```python
from build123d import *

# Parameters (mm, degrees)
SKETCH1_R               = 22
SKETCH1_R_2             = 20
BOSS_EXTRUDE1_DEPTH     = 40
CUT_EXTRUDE1_DEPTH      = 23
CUT_EXTRUDE1_DEPTH_BACK = 23
BOSS_EXTRUDE2_DEPTH     = 20
SKETCH4_W               = 28
SKETCH4_H               = 39
CUT_EXTRUDE2_DEPTH      = 32
SKETCH5_R               = 3.5
CUT_EXTRUDE3_DEPTH      = 8.79196205
CUT_EXTRUDE3_DEPTH_BACK = 37.20803795
FILLET1_R               = 8


with BuildPart() as part:
    # Sketch1 → Boss-Extrude1 (new body)
    with BuildSketch(Plane(origin=(0, 0, 0), x_dir=(1, 0, 0), z_dir=(0, 1, 0))):
        Circle(SKETCH1_R)
        Circle(SKETCH1_R_2, mode=Mode.SUBTRACT)
    extrude(amount=BOSS_EXTRUDE1_DEPTH)

    # Sketch2 → Cut-Extrude1 (cut, two sides)
    with BuildSketch(Plane.XY) as cut_extrude1_sk:
        Polygon((22, 33), (-22, 0), (22, 0), align=None)
    extrude(amount=CUT_EXTRUDE1_DEPTH, mode=Mode.SUBTRACT)
    extrude(cut_extrude1_sk.sketch, amount=-CUT_EXTRUDE1_DEPTH_BACK, mode=Mode.SUBTRACT)

    # Sketch3 → Boss-Extrude2 (add)
    with BuildSketch(Plane(origin=(-31, 0, 0), x_dir=(0, 0, -1), z_dir=(1, 0, 0))):
        Polygon((14.20803795, 40), (-17.79196205, 40), (-17.79196205, -1), (-15.79196205, -1), (-15.79196205, 1), (-15.79196205, 38), (12.20803795, 38), (12.20803795, 1), (12.20803795, -1), (14.20803795, -1), align=None)
    extrude(amount=BOSS_EXTRUDE2_DEPTH)

    # Sketch4 → Cut-Extrude2 (cut, through all)
    with BuildSketch(Plane(origin=(0, 0, 0), x_dir=(0, 0, -1), z_dir=(1, 0, 0))):
        with Locations((-1.79196205, 18.5)):
            Rectangle(SKETCH4_W, SKETCH4_H)
    extrude(amount=-CUT_EXTRUDE2_DEPTH, mode=Mode.SUBTRACT)

    # Sketch5 → Cut-Extrude3 (cut, two sides)
    with BuildSketch(Plane(origin=(0, 0, -14.20803795), x_dir=(-1, 0, 0), z_dir=(0, 0, -1))) as cut_extrude3_sk:
        with Locations((24, 6)):
            Circle(SKETCH5_R)
    extrude(amount=CUT_EXTRUDE3_DEPTH, mode=Mode.SUBTRACT)
    extrude(cut_extrude3_sk.sketch, amount=-CUT_EXTRUDE3_DEPTH_BACK, mode=Mode.SUBTRACT)

    # Fillet1
    fillet1_edges = [part.edges().sort_by_distance(p)[0] for p in [
        (-11, -1, 16.79196205),
        (-11, -1, -13.20803795),
    ]]
    fillet(fillet1_edges, radius=FILLET1_R)


solid = part.part
```
Verification items for the finished model (mm, model axes). A direction names the side the tool comes from. Round coordinates to 2 decimals unless told otherwise and drop trailing zeros. Order: outer loops, then holes, each group sorted by start corner. A loop starts at its lowest first (then second) coordinate and runs counter-clockwise, first axis right, second up.
1) Cross-section at A-A, the plane x = 0. Record the cut outline in (y, z), plus the area to 3 significant figures.
Geometry says:
outline: (16.5, -22) - (40, -22) - (40, -20) - (16.5, -20) - close; (16.5, 20) - (40, 20) - (40, 22) - (16.5, 22) - close
area: 94.0 mm2
2) Draft check along Y on faces 1 (the flat face through (-14, 40, 2)), 2 (the cylindrical face through (-25.615, 2.895, 16.778)), 3 (the flat face through (-25, -1, -13)). Enter one of: +Y half, -Y half, draft (parallel to the pull), parting line (faces both ways), or undercut.
Geometry says:
face 1: +Y half
face 2: undercut
face 3: -Y half
3) Cross-section at B-B, the plane x = -24. Record the cut outline in (y, z).
Geometry says:
outline: (-1, -14.21) - (2.5, -14.21) - (2.5, -12.21) - (-1, -12.21) - close; (-1, 15.79) - (2.5, 15.79) - (2.5, 17.79) - (-1, 17.79) - close; (9.5, -14.21) - (40, -14.21) - (40, 17.79) - (9.5, 17.79) - (9.5, 15.79) - (38, 15.79) - (38, -12.21) - (9.5, -12.21) - close
4) Cross-section at D-D, the plane z = -6. Record the cut outline in (x, y), plus the area to 3 significant figures.
Geometry says:
outline: (-31, 38) - (-11, 38) - (-11, 40) - (-31, 40) - close; (19.08, 30.81) - (21.17, 32.37) - (21.17, 40) - (19.08, 40) - close
area: 57.5 mm2
5) Cross-section at C-C, the plane y = 11. Record the cut outline in (x, z), plus the area to 3 significant figures.
Geometry says:
outline: (-31, -14.21) - (-16.8, -14.21) arc R22 ccw to (-7.33, -20.74) - (-7.33, -18.61) arc R20 cw to (-14.08, -14.21) - (-11, -14.21) - (-11, -12.21) - (-31, -12.21) - close; (-31, 15.79) - (-11, 15.79) - (-11, 16.7) arc R20 cw to (-7.33, 18.61) - (-7.33, 20.74) arc R22 ccw to (-12.94, 17.79) - (-31, 17.79) - close
area: 109 mm2
6) Tool access check on faces 4 (the flat face through (-21, 18, 15.792)), 5 (the cylindrical face through (-13.281, 1.406, -13.222)). Record the directions out of +Z, -Z, +X, -X, +Y, -Y that give a thin tool (end or side, any length) a straight path to the whole face; none if there is none.
Geometry says:
face 4: -X, -Y
face 5: +Z, -Z, +X, -Y
7) Material ranges on line 1 (Y direction, x = -24, z = -13.75); line 2 (Z direction, x = -21, y = 27.5); line 3 (Z direction, x = 0, y = 21), recorded low to high.
Geometry says:
line 1: y = -1 to 2.5, 9.5 to 40
line 2: z = -14.21 to -12.21, 15.79 to 17.79
line 3: z = -22 to -20, 20 to 22
8) Depth check by flat-ended pin: pin 1 (22 mm diameter, centred on x = -16.5, y = 16, fed in from +Z); pin 2 (6 mm diameter, centred on x = -25, y = 28.5, fed in from -Z); pin 3 (22 mm diameter, centred on x = -23.5, y = 14.5, fed in from +Z); pin 4 (8 mm diameter, centred on y = 23.5, z = 5.5, fed in from +X). Enter the tip coordinate at first touch or a pass-through.
Geometry says:
pin 1: stops at z = 21.3
pin 2: stops at z = -14.21
pin 3: stops at z = 18.1
pin 4: passes through
